Design review of the part built by this model. Coordinates are the model's own, in mm. Face numbers are marked on the shaded views. A direction names the side the tool comes from. Round coordinates to 2 decimals unless told otherwise and drop trailing zeros. Loops run counter-clockwise (first coordinate to the right, second up) from the corner with the lowest first, then second, coordinate; pieces in that order, holes last. Notation, with made-up numbers: (25, 11.5) - (68, 11.5) arc R28 ccw to (68, 49.5) - close; hole circle Ø2 at (5, 69). An arc over 180 degrees is marked (long way). Use one line per item in the form item = value. Start each with the question number.
(1) For pin 1 (0.9 mm diameter, centred on y = 30.5, z = 2, fed in from +X); pin 2 (2.5 mm diameter, centred on x = 68, z = 1, fed in from -Y); pin 3 (3 mm diameter, centred on x = 17.5, z = 41.5, fed in from -Y), all flat-tipped, find the tip position at first contact; note any pin that passes through.
(2) The part is to be moulded in two halves that separate along Z. For the marked faces 3, 4 and 5, say which applies: released by +Z, released by -Z, zero draft, split by the parting line, or undercut.
(3) Machinability: for the marked faces 1 and 2, which of the approach directions +Z, -Z, +X, -X, +Y, -Y give a long, thin tool a straight path to every point of the face, cutting with its end or side? Answer none if there is none.
(4) Wall thickness on probe 1 along Z at (x, y) = (90.5, 93); probe 2 along Y at (x, z) = (89.5, 22); probe 3 along X at (y, z) = (70, 42.5): over which ranges is each line inside the solid? List them lowest first. Write a range as [from, to].
(5) We need section A-A, the plane x = 12.5. Write out the cut boundary in (y, z).
(6) We need section C-C, the plane z = 29. Write out the cut boundary in (x, y), then the cut area to 3 significant figures.
(7) We need section B-B, the plane y = 40.5. Write out the cut boundary in (x, z).
from build123d import *

# Parameters (mm, degrees)
LINEAR_AUSTRAGEN_D_NN1_DEPTH    = 50
SKIZZE3_W                       = 44
SKIZZE3_H                       = 100.666411599
SCHNITT_LINEAR_AUSTRAGEN2_DEPTH = 97


with BuildPart() as part:
    # Skizze1 → Linear-Austragen-Dünn1 (new body)
    with BuildSketch(Plane.XY):
        Polygon((0, 0), (0, 100), (100, 100), (100, 85), (15, 85), (15, 0), align=None)
    extrude(amount=LINEAR_AUSTRAGEN_D_NN1_DEPTH)

    # Skizze3 → Schnitt-Linear austragen2 (cut)
    with BuildSketch(Plane(origin=(100, 0, 0), x_dir=(0, 0, -1), z_dir=(1, 0, 0))):
        with Locations((-25, 46.666794201)):
            Rectangle(SKIZZE3_W, SKIZZE3_H)
    extrude(amount=-SCHNITT_LINEAR_AUSTRAGEN2_DEPTH, mode=Mode.SUBTRACT)


solid = part.part
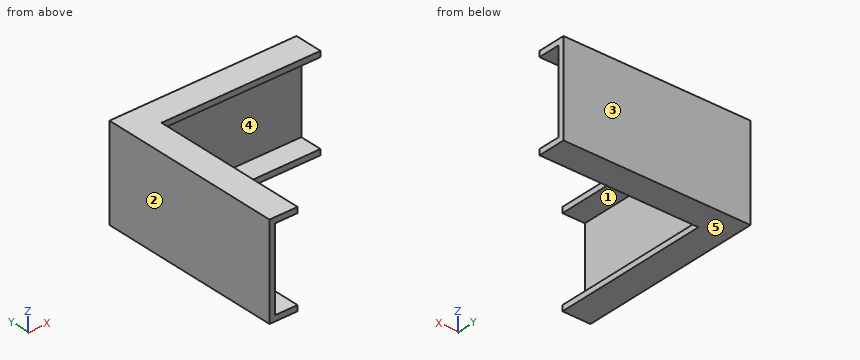
Data:
q1.pin_1 = 15
q1.pin_2 = 85
q1.pin_3 = 97
q2.face_3 = zero draft
q2.face_4 = undercut
q2.face_5 = released by -Z
q3.face_1 = +X, -Y
q3.face_2 = +Z, -Z, -X, +Y, -Y
q4.probe_1 = [0, 3], [47, 50]
q4.probe_2 = [97, 100]
q4.probe_3 = [0, 3]
q5.outline = (0, 0) - (100, 0) - (100, 50) - (0, 50) - (0, 47) - (97, 47) - (97, 3) - (0, 3) - close
q6.outline = (0, 0) - (3, 0) - (3, 97) - (100, 97) - (100, 100) - (0, 100) - close
q6.area = 591 mm^2
q7.outline = (0, 0) - (15, 0) - (15, 3) - (3, 3) - (3, 47) - (15, 47) - (15, 50) - (0, 50) - close
